Read the model definition and answer for the solid it produces. Units are mm, in the model's axes. Face numbers are marked on the shaded views. A direction names the side the tool comes from. Round coordinates to 2 decimals unless told otherwise and drop trailing zeros. Loops run counter-clockwise (first coordinate to the right, second up) from the corner with the lowest first, then second, coordinate; pieces in that order, holes last. Notation, with made-up numbers: M -14.75,61 L 25.25,61 A16 cw 25.25,90 Z; hole C 27.5,16.5 d1. An arc over 180 degrees is marked long. Answer as CSV lines item,"result".
```python
from build123d import *

# Parameters (mm, degrees)
SALIENTE_EXTRUIR1_DEPTH = 5
CROQUIS2_W              = 5
CROQUIS2_H              = 90
SALIENTE_EXTRUIR2_DEPTH = 60
CORTAR_EXTRUIR1_DEPTH   = 5
SALIENTE_EXTRUIR3_DEPTH = 5
REDONDEO1_R             = 3
CROQUIS5_W              = 58
CROQUIS5_H              = 5
SALIENTE_EXTRUIR4_DEPTH = 60
CORTAR_EXTRUIR2_DEPTH   = 5
REDONDEO2_R             = 3
REDONDEO3_R             = 3
CROQUIS7_R              = 1.75
CROQUIS7_R_2            = 3.15
CORTAR_EXTRUIR3_DEPTH   = 5


with BuildPart() as part:
    # Croquis1 → Saliente-Extruir1 (new body)
    with BuildSketch(Plane.XY):
        with BuildLine():
            Line((-63, 0), (0, 0))
            Line((0, 0), (0, -90))
            Line((0, -90), (-33, -90))
            Line((-33, -90), (-33, -48))
            ThreePointArc((-33, -48), (-41.786797, -26.786797), (-63, -18))
            Line((-63, -18), (-63, 0))
        make_face()
    extrude(amount=SALIENTE_EXTRUIR1_DEPTH)

    # Croquis2 → Saliente-Extruir2 (add)
    with BuildSketch(Plane.XY.offset(5)):
        with Locations((-2.5, -45)):
            Rectangle(CROQUIS2_W, CROQUIS2_H)
    extrude(amount=SALIENTE_EXTRUIR2_DEPTH)

    # Croquis3 → Cortar-Extruir1 (cut)
    with BuildSketch(Plane(origin=(0, 0, 0), x_dir=(0, 0, -1), z_dir=(1, 0, 0))):
        with BuildLine():
            Line((-65, -90), (-35, -90))
            Line((-35, -90), (-35, -48))
            ThreePointArc((-35, -48), (-43.786797, -26.786797), (-65, -18))
            Line((-65, -18), (-65, -90))
        make_face()
    extrude(amount=-CORTAR_EXTRUIR1_DEPTH, mode=Mode.SUBTRACT)

    # Croquis4 → Saliente-Extruir3 (add)
    with BuildSketch(Plane.XZ.offset(90)):
        Polygon((-33, 8), (-8, 8), (-8, 35), (-5, 35), (-5, 5), (-33, 5), align=None)
    extrude(amount=-SALIENTE_EXTRUIR3_DEPTH)

    # Redondeo1
    redondeo1_edges = [part.edges().sort_by_distance(p)[0] for p in [
        (-33, -87.5, 8),
        (-8, -87.5, 35),
    ]]
    fillet(redondeo1_edges, radius=REDONDEO1_R)

    # Croquis5 → Saliente-Extruir4 (add)
    with BuildSketch(Plane.XY.offset(5)):
        with Locations((-34, -12.5)):
            Rectangle(CROQUIS5_W, CROQUIS5_H)
    extrude(amount=SALIENTE_EXTRUIR4_DEPTH)

    # Croquis6 → Cortar-Extruir2 (cut)
    with BuildSketch(Plane(origin=(0, -10, 0), x_dir=(1, 0, 0), z_dir=(0, 1, 0))):
        Polygon((-63, -19.817641), (-17.817641, -65), (-63, -65), align=None)
    extrude(amount=-CORTAR_EXTRUIR2_DEPTH, mode=Mode.SUBTRACT)

    # Redondeo2
    redondeo2_edges = [part.edges().sort_by_distance(p)[0] for p in [
        (-63, -12.5, 19.817641),
        (-17.817641, -12.5, 65),
    ]]
    fillet(redondeo2_edges, radius=REDONDEO2_R)

    # Redondeo3
    redondeo3_edges = [part.edges().sort_by_distance(p)[0] for p in [
        (-34, -15, 5),
        (-5, -15, 35),
        (-5, -50, 5),
    ]]
    fillet(redondeo3_edges, radius=REDONDEO3_R)

    # Croquis7 → Cortar-Extruir3 (cut)
    with BuildSketch(Plane(origin=(0, -10, 0), x_dir=(1, 0, 0), z_dir=(0, 1, 0))):
        with Locations((-15, -55)):
            Circle(CROQUIS7_R)
        with Locations((-15, -15)):
            Circle(CROQUIS7_R)
        with Locations((-55, -15)):
            Circle(CROQUIS7_R)
        with Locations((-29.5, -24.5)):
            Circle(CROQUIS7_R_2)
    extrude(amount=-CORTAR_EXTRUIR3_DEPTH, mode=Mode.SUBTRACT)


solid = part.part
```
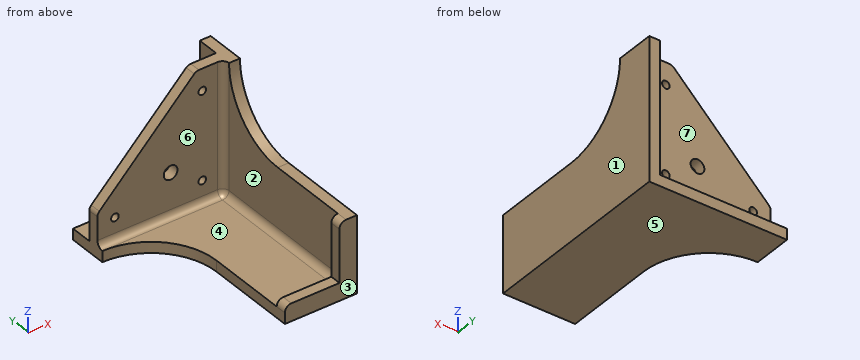
1) Each of these flat-tipped pins is pushed along its axis until it touches: P1, Ø1.5, axis at x = -40, z = 11, coming from the +Y side; P2, Ø5, axis at y = -3, z = 36, coming from the -X side; P3, Ø1.5, axis at x = -15.5, y = -88.5, coming from the +Z side; P4, Ø3, axis at x = -55, z = 15, coming from the +Y side. Where does it stop, or does it pass through?
Evaluation:
P1,"stops at y = -10"
P2,"stops at x = -5"
P3,"stops at z = 8"
P4,"passes through"
2) Find section A-A, the plane x = -15. Give the vertices of the cut face in (y, z), then the cut area to 3 significant figures.
Evaluation:
outline,"M -90,0 L 0,0 L 0,5 L -10,5 L -10,13.25 L -15,13.25 L -15,8 A3 cw -18,5 L -85,5 L -85,8 L -90,8 Z; M -15,16.75 L -10,16.75 L -10,53.25 L -15,53.25 Z; M -15,56.75 L -10,56.75 L -10,65 L -15,65 Z"
area,"732 mm^2"
3) Find section C-C, the plane y = -68. Give the vertices of the cut face in (x, z), then the cut area to 3 significant figures.
Evaluation:
outline,"M -33,0 L 0,0 L 0,35 L -5,35 L -5,8 A3 cw -8,5 L -33,5 Z"
area,"317 mm^2"
4) Find section D-D, the plane z = 24.5. Give the vertices of the cut face in (x, y), then the cut area to 3 significant figures.
Evaluation:
outline,"M -58.32,-15 L -32.65,-15 L -32.65,-10 L -58.32,-10 Z; M -26.35,-15 L -8,-15 A3 cw -5,-18 L -5,-85 L -8,-85 L -8,-90 L 0,-90 L 0,0 L -5,0 L -5,-10 L -26.35,-10 Z"
area,"702 mm^2"
5) Find section B-B, the plane z = 15. Give the vertices of the cut face in (x, y).
Evaluation:
outline,"M -63,-15 L -56.75,-15 L -56.75,-10 L -63,-10 Z; M -53.25,-15 L -16.75,-15 L -16.75,-10 L -53.25,-10 Z; M -13.25,-15 L -8,-15 A3 cw -5,-18 L -5,-85 L -8,-85 L -8,-90 L 0,-90 L 0,0 L -5,0 L -5,-10 L -13.25,-10 Z"
6) Straight lines are drawn through the part: line 1 (Z direction, x = -15, y = -13.75); line 2 (X direction, y = -11.75, z = 15); line 3 (Y direction, x = -12.5, z = 36.5). For each, find the intervals that lie inside material, in ascending order.
Evaluation:
line 1,"z = 0 to 13.25, 16.75 to 53.25, 56.75 to 65"
line 2,"x = -63 to -56.75, -53.25 to -16.75, -13.25 to 0"
line 3,"y = -15 to -10"
7) Determine the mould class of the marked faces 1, 2 and 3 for opening direction Y: released by +Y, released by -Y, zero draft, split by the parting line, or undercut.
Evaluation:
face 1,"zero draft"
face 2,"undercut"
face 3,"released by -Y"
8) A tool of negligible diameter and unlimited length cuts with its end or side. For the marked faces 4, 5, 6 and 7, from which of +Z, -Z, +X, -X, +Y, -Y can it reach the whole face along a straight path? Write none if from no direction.
Evaluation:
face 4,"+Z, -X"
face 5,"-Z, +X, -X, +Y, -Y"
face 6,"+Z, -X, -Y"
face 7,"+Z, -X, +Y"
